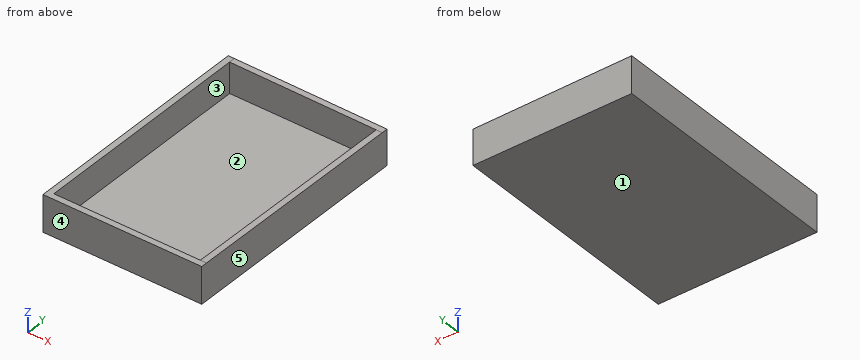
```python
from build123d import *

# Parameters (mm, degrees)
F0_W     = 132.08
F0_H     = 198.12
F1_DEPTH = 5.08
F2_W     = 132.08
F2_H     = 25.4
F3_DEPTH = 5.08
F4_W     = 193.04
F4_H     = 25.4
F5_DEPTH = 5.08
F7_DEPTH = 5.08
F9_DEPTH = 5.08


with BuildPart() as f1:
    # F0 (on Top) → F1 (new body)
    with BuildSketch(Plane.XY):
        with Locations((-10.161369, 9.438567)):
            Rectangle(F0_W, F0_H)
    extrude(amount=F1_DEPTH)

    # F2 (on face) → F3 (join)
    with BuildSketch(Plane.XZ.offset(89.621433)):
        with Locations((-10.161369, 17.78)):
            Rectangle(F2_W, F2_H)
    extrude(amount=-F3_DEPTH)

    # F4 (on face) → F5 (join)
    with BuildSketch(Plane(origin=(-76.201369, 0, 0), x_dir=(0, -1, 0), z_dir=(-1, 0, 0))):
        with Locations((-11.978567, 17.78)):
            Rectangle(F4_W, F4_H)
    extrude(amount=-F5_DEPTH)

    # F6 (on face) → F7 (join)
    with BuildSketch(Plane(origin=(0, 108.498567, 0), x_dir=(-1, 0, 0), z_dir=(0, 1, 0))):
        Polygon((-55.878631, 29.360438), (-55.878631, 5.08), (71.121369, 5.08), (71.121369, 30.48), align=None)
    extrude(amount=-F7_DEPTH)

    # F8 (on face) → F9 (join)
    with BuildSketch(Plane.YZ.offset(55.878631)):
        Polygon((103.418567, 29.360438), (-84.541433, 30.48), (-84.541433, 5.08), (103.418567, 5.08), align=None)
    extrude(amount=-F9_DEPTH)


solid = f1.part
```
Could you check a few things on this model? Use its own coordinates, in mm. Face numbers are marked on the shaded views. A direction names the side the tool comes from. Round coordinates to 2 decimals unless told otherwise and drop trailing zeros. Loops run counter-clockwise (first coordinate to the right, second up) from the corner with the lowest first, then second, coordinate; pieces in that order, holes last. Notation, with made-up numbers: (50, 44.25) -> (56, 44.25) arc R13 cw to (56, 50.25) -> close; hole circle Ø6 at (70, 69.25). An arc over 180 degrees is marked (long way). One line per question, with ' | ' between items.
(1) If we section it at C-C on y = 24: List the corners of the cut face in (x, z) for me.
Model answer:
outline: (-76.2, 0) -> (55.88, 0) -> (55.88, 29.83) -> (50.8, 29.83) -> (50.8, 5.08) -> (-71.12, 5.08) -> (-71.12, 30.48) -> (-76.2, 30.48) -> close
(2) If I drill on probe 1 along X at (y, z) = (-33.5, 17); probe 2 along Y at (x, z) = (-63, 25.5); probe 3 along Z at (x, y) = (-51, 2), over which ranges is the centre line in solid material (lowest first)?
Model answer:
probe 1: x = -76.2 to -71.12, 50.8 to 55.88 | probe 2: y = -89.62 to -84.54, 103.42 to 108.5 | probe 3: z = 0 to 5.08
(3) Thinking about a two-plate mould opening in X: for the marked faces 3, 4 and 5, which applies, released by +X, released by -X, zero draft, split by the parting line, or undercut?
Model answer:
face 3: undercut | face 4: zero draft | face 5: released by +X
(4) For pin 1 Ø1.5 at (x, y) = (18, 75) entering from +Z, with a flat end and sliding along its axis, tell me the tip position at first contact or that it passes through.
Model answer:
pin 1: stops at z = 5.08
(5) If we section it at A-A on z = 9: List the corners of the cut face in (x, y) for me, and give its area (3 significant figures).
Model answer:
outline: (-76.2, -89.62) -> (55.88, -89.62) -> (55.88, 108.5) -> (-76.2, 108.5) -> close; hole (-71.12, -84.54) -> (50.8, -84.54) -> (50.8, 103.42) -> (-71.12, 103.42) -> close | area: 3,250 mm^2
(6) If we section it at B-B on x = -32.5: List the corners of the cut face in (y, z) for me.
Model answer:
outline: (-89.62, 0) -> (108.5, 0) -> (108.5, 30.14) -> (103.42, 30.14) -> (103.42, 5.08) -> (-84.54, 5.08) -> (-84.54, 30.48) -> (-89.62, 30.48) -> close
(7) For the marked faces 1 and 2, which set-ups out of +Z, -Z, +X, -X, +Y, -Y let a thin tool reach every point of the face, with its end or its side?
Model answer:
face 1: -Z, +X, -X, +Y, -Y | face 2: +Z
